Read the model definition and answer for the solid it produces. Units are mm, in the model's axes. A direction names the side the tool comes from. Coordinates: 2 decimals unless noted, no trailing zeros. Order: outer loops, then holes, each group sorted by start corner. A loop starts at its lowest first (then second) coordinate and runs counter-clockwise, first axis right, second up. Notation, with made-up numbers: (83.5, 31.5) - (140.5, 31.5) arc R27 ccw to (140.5, 69.5) - close; hole circle Ø10 at (-20.5, 83). An arc over 180 degrees is marked (long way). Write item = value, one per line.
from build123d import *

# Parameters (mm, degrees)
BOSS_EXTRU_1_DEPTH      = 3
BOSS_EXTRU_2_START      = -3
ESQUISSE2_W             = 33.166247904
ESQUISSE2_H             = 3
BOSS_EXTRU_2_DEPTH      = 10
ENL_V_MAT_EXTRU_1_DEPTH = 64.984373092
ESQUISSE4_R             = 1.5
ENL_V_MAT_EXTRU_2_DEPTH = 62.424750712


with BuildPart() as part:
    # Esquisse1 → Boss.-Extru.1 (new body)
    with BuildSketch(Plane.XY):
        with BuildLine():
            Line((16.583123952, 25), (-16.583123952, 25))
            ThreePointArc((-16.583123952, 25), (-14.186371655, -26.433820369), (30, 0))
            ThreePointArc((30, 0), (26.433820369, 14.186371655), (16.583123952, 25))
        make_face()
    extrude(amount=BOSS_EXTRU_1_DEPTH)

    # Esquisse2 → Boss.-Extru.2 (add)
    with BuildSketch(Plane(origin=(0, 0, 0), x_dir=(-1, 0, 0), z_dir=(0, 0, -1)).offset(BOSS_EXTRU_2_START)):
        with Locations((0, 23.5)):
            Rectangle(ESQUISSE2_W, ESQUISSE2_H)
    extrude(amount=-BOSS_EXTRU_2_DEPTH)

    # Esquisse3 → Enlèv. mat.-Extru.1 (cut, through all)
    with BuildSketch(Plane(origin=(0, 25, 0), x_dir=(1, 0, 0), z_dir=(0, 1, 0))):
        with BuildLine():
            Line((11.024660406, -13), (16.583123952, -13))
            Line((16.583123952, -13), (16.583123952, -8.593951902))
            ThreePointArc((16.583123952, -8.593951902), (13.978605431, -11.017385992), (11.024660406, -13))
        make_face()
        with BuildLine():
            Line((-16.583123952, -8.589860243), (-16.583123952, -13))
            Line((-16.583123952, -13), (-11.02090831, -13))
            ThreePointArc((-11.02090831, -13), (-13.977028503, -11.015661574), (-16.583123952, -8.589860243))
        make_face()
    extrude(amount=-ENL_V_MAT_EXTRU_1_DEPTH, mode=Mode.SUBTRACT)

    # Esquisse4 → Enlèv. mat.-Extru.2 (cut, through all)
    with BuildSketch(Plane.XZ.offset(-22)):
        with Locations(Location((-9.833123952, 9, 0), (0, 0, 270))):
            Circle(ESQUISSE4_R)
        with Locations(Location((9.833123952, 9, 0), (0, 0, 90))):
            Circle(ESQUISSE4_R)
    extrude(amount=-ENL_V_MAT_EXTRU_2_DEPTH, mode=Mode.SUBTRACT)


solid = part.part
1) The part is cut by section A-A (z = 4). Determine the outline of the cut face in (x, y).
Returned:
outline = (-16.58, 22) - (16.58, 22) - (16.58, 25) - (-16.58, 25) - close
2) The part is cut by section C-C (y = 9). Determine the outline of the cut face in (x, z), and give its area (3 significant figures).
Returned:
outline = (-28.62, 0) - (28.62, 0) - (28.62, 3) - (-28.62, 3) - close
area = 172 mm^2
3) Straight lines are drawn through the part: line 1 along X through (y, z) = (23.2, 9); line 2 along Z through (x, y) = (-21.5, -5.5); line 3 along X through (y, z) = (14.5, 2.75). For each, find the intervals that lie inside material, in ascending order. Write a range as from..to.
Returned:
line_1 = -16.2..-11.33, -8.33..8.33, 11.33..16.2
line_2 = 0..3
line_3 = -26.26..26.26
4) Determine the mould class of faces 1 (the face through (-13.938, 23.521, 11.047)), 2 (the face through (8.819, 23.479, 7.894)), 3 (the face through (14, 24, 11)) for opening direction X: pulls with the +X half, pulls with the -X half, needs draft (parallel to the pull), parting line crosses it, or undercut.
Returned:
face_1 = pulls with the -X half
face_2 = undercut
face_3 = pulls with the +X half
5) For faces 4 (the face through (16.583, 23, 6)), 5 (the face through (-16.583, 23, 6)), 6 (the face through (0, 22, 8)), determine the directions among +Z, -Z, +X, -X, +Y, -Y from which every point of the face is accessible in a straight line to the end or side of a thin tool.
Returned:
face_4 = +Z, +X, +Y, -Y
face_5 = +Z, -X, +Y, -Y
face_6 = +Z, +X, -X, -Y
6) Flat-ended cylindrical pins translate along their axes: pin 1 Ø2.5 at (x, z) = (-9.83, 9) entering from +Y; pin 2 Ø5 at (y, z) = (4, 2.5) entering from +X; pin 3 Ø3.5 at (y, z) = (23, 5) entering from -X; pin 4 Ø3 at (x, z) = (-7, 10.5) entering from -Y. Find the tip coordinate at first contact, or state that the pin passes through.
Returned:
pin_1 = through
pin_2 = 29.96
pin_3 = -16.58
pin_4 = 22
7) The part is cut by section B-B (x = 0). Determine the outline of the cut face in (y, z), and give its area (3 significant figures).
Returned:
outline = (-30, 0) - (25, 0) - (25, 13) - (22, 13) - (22, 3) - (-30, 3) - close
area = 195 mm^2
8) The part is cut by section D-D (x = -14). Determine the outline of the cut face in (y, z).
Returned:
outline = (-26.53, 0) - (25, 0) - (25, 11) - (22, 11) - (22, 3) - (-26.53, 3) - close
